Job drawing, mm, ordinate dimensions from the low corner. One solid piece. A direction names the side the tool comes from. Round coordinates to 2 decimals unless told otherwise and drop trailing zeros. Loops run counter-clockwise (first coordinate to the right, second up) from the corner with the lowest first, then second, coordinate; pieces in that order, holes last. Notation, with made-up numbers: (57, 18.25) - (89, 18.25) arc R5 ccw to (89, 25.25) - close; hole circle Ø10 at (-12.5, 0.25). An arc over 180 degrees is marked (long way). One line per question, with ' | ' between items. Start each with the question number.
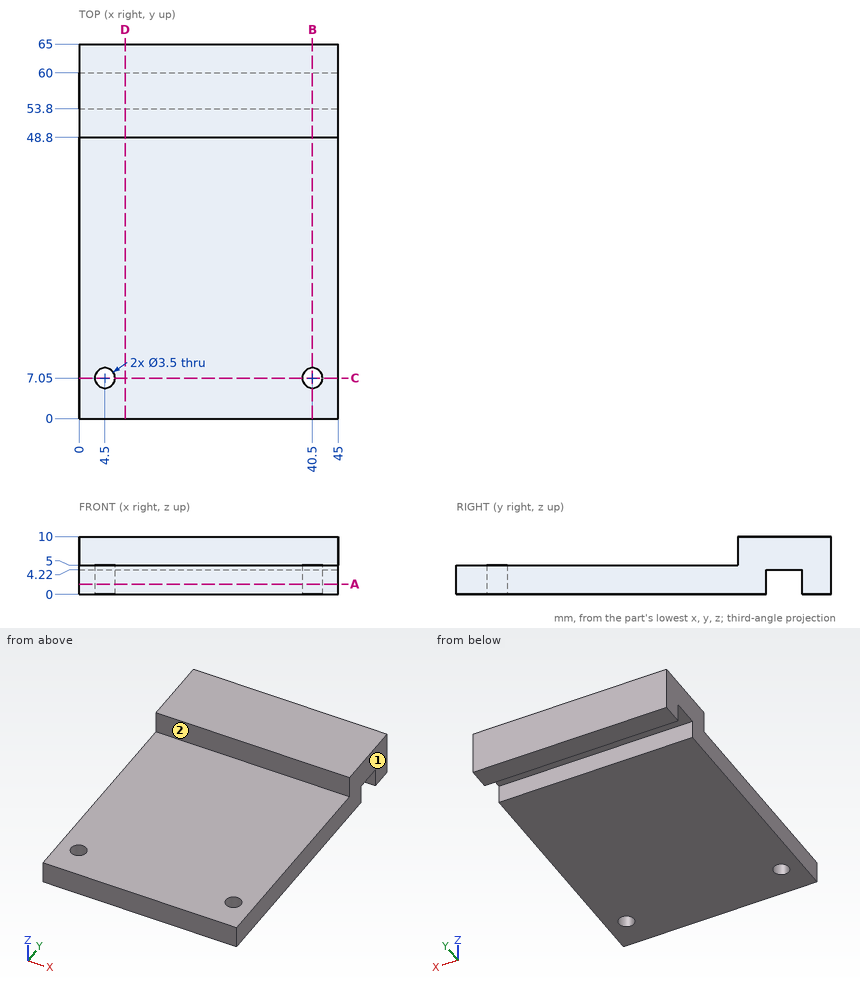
1) Tool access for the marked faces 1 and 2: list every direction of +Z, -Z, +X, -X, +Y, -Y with a clear straight run to the whole face (end or side of a thin tool).
2) Saw through at C-C on y = 7.05. Write the cut outline in (x, z), and give its area (3 significant figures).
3) Wall check: line 1 (Y direction, x = 40.5, z = 2.55); line 2 (Y direction, x = 4, z = 3); line 3 (Z direction, x = 6.5, y = 46.5). Give the ranges that are in metal, low to high. Write a range as [from, to].
4) Drop flat-ended pins along their axis: pin 1 (1.3 mm diameter, centred on x = 28.5, z = 2, fed in from -Y); pin 2 (1.9 mm diameter, centred on x = 26.5, y = 57.5, fed in from -Z); pin 3 (5 mm diameter, centred on x = 31, y = 22, fed in from +Z); pin 4 (1.5 mm diameter, centred on x = 17, z = 8.5, fed in from -Y). Give the stop position or say it passes through.
5) Saw through at A-A on z = 1.75. Write the cut outline in (x, y), and give its area (3 significant figures).
6) Saw through at B-B on x = 40.5. Write the cut outline in (y, z), and give its area (3 significant figures).
7) Saw through at D-D on x = 8. Write the cut outline in (y, z), and give its area (3 significant figures).
Answer key:
1) face 1: +Z, -Z, +X, +Y, -Y | face 2: +Z, +X, -X, -Y
2) outline: (0, 0) - (2.75, 0) - (2.75, 5) - (0, 5) - close; (6.25, 0) - (38.75, 0) - (38.75, 5) - (6.25, 5) - close; (42.25, 0) - (45, 0) - (45, 5) - (42.25, 5) - close | area: 190 mm²
3) line 1: [0, 5.3], [8.8, 53.8], [60, 65] | line 2: [0, 5.37], [8.73, 53.8], [60, 65] | line 3: [0, 5]
4) pin 1: y = 0 | pin 2: z = 4.22 | pin 3: z = 5 | pin 4: y = 48.8
5) outline: (0, 0) - (45, 0) - (45, 53.8) - (0, 53.8) - close; (0, 60) - (45, 60) - (45, 65) - (0, 65) - close; hole circle Ø3.5 at (4.5, 7.05); hole circle Ø3.5 at (40.5, 7.05) | area: 2,630 mm²
6) outline: (0, 0) - (5.3, 0) - (5.3, 5) - (0, 5) - close; (8.8, 0) - (53.8, 0) - (53.8, 4.22) - (60, 4.22) - (60, 0) - (65, 0) - (65, 10) - (48.8, 10) - (48.8, 5) - (8.8, 5) - close | area: 362 mm²
7) outline: (0, 0) - (53.8, 0) - (53.8, 4.22) - (60, 4.22) - (60, 0) - (65, 0) - (65, 10) - (48.8, 10) - (48.8, 5) - (0, 5) - close | area: 380 mm²
